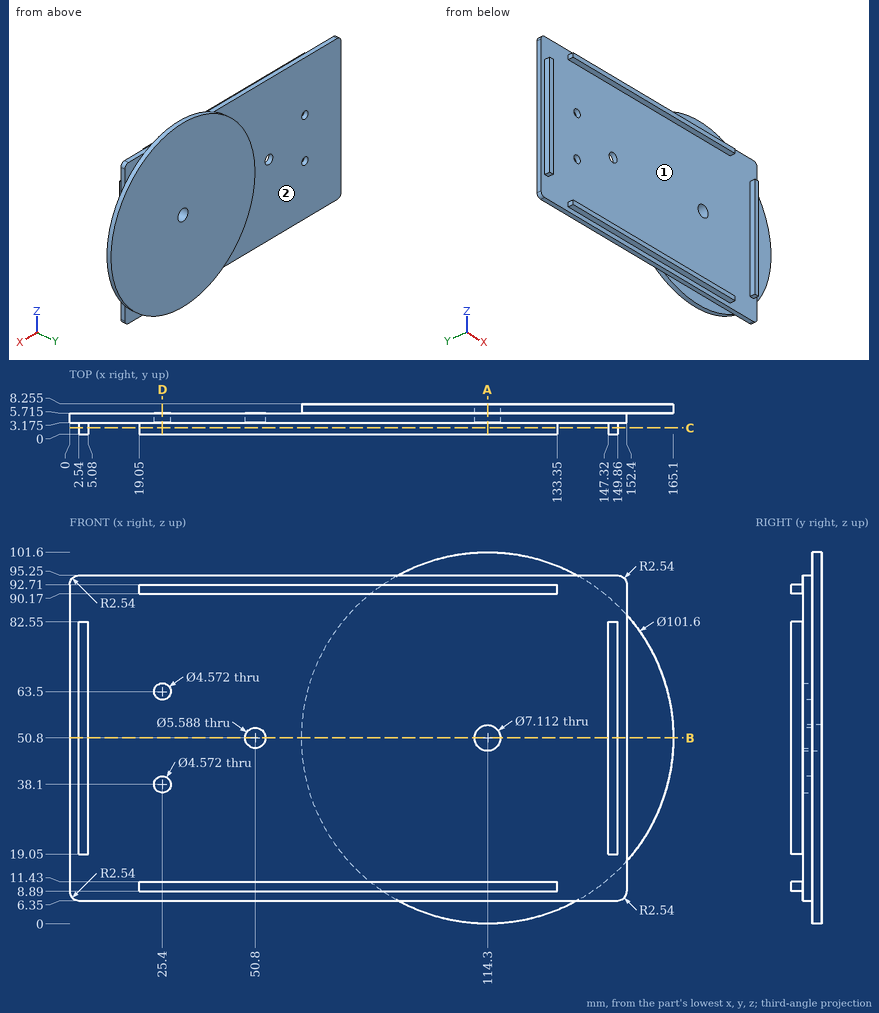
Print and shaded views of the part. All mm, measured from the part's lowest x, y and z. Round coordinates to 2 decimals unless told otherwise and drop trailing zeros. Write each loop counter-clockwise with the first axis right and the second up, starting at its lowest first coordinate (ties: lowest second). Pieces come first, ordered by that corner, then holes. Notation, with made-up numbers: (-15.75, 12.5) -> (8.25, 12.5) arc R22 ccw to (8.25, 39.5) -> close; hole circle Ø9 at (-5, -37.5). An arc over 180 degrees is marked (long way). Return JSON: item names as keys, results as strings. Group by question number.
Q1. Mould opens along Z. For the marked faces 1 and 2 say: pulls with the +Z half, pulls with the -Z half, needs draft (parallel to the pull), parting line crosses it, or undercut.
Q2. Saw through at C-C on y = 1.75. Write the cut outline in (x, z).
Q3. Probe L1, parallel to X at y = 4.25, z = 50.8; L2, parallel to Z at x = 31, y = 1.75; L3, parallel to X at y = 4.85, z = 38.1. List the from-to ranges inside material, lowest first. Write a range as [from, to].
Q4. Pin check, flat tips, straight feed: pin 1 (0.8 mm diameter, centred on y = 5, z = 52.5, fed in from +X); pin 2 (0.8 mm diameter, centred on x = 4, y = 1, fed in from +Z); pin 3 (4.5 mm diameter, centred on x = 114.3, z = 50.8, fed in from +Y); pin 4 (2 mm diameter, centred on x = 18.5, z = 34.5, fed in from +Y) (3 decimals). Stop position of each tip, or through.
Q5. Saw through at D-D on x = 25.4. Write the cut outline in (y, z) (3 decimals), plus the area to 3 significant figures.
Q6. Saw through at B-B on z = 50.8. Write the cut outline in (x, y) (3 decimals), plus the area to 3 significant figures.
Q7. Saw through at A-A on x = 114.3. Write the cut outline in (y, z) (3 decimals).
Answer:
{
 "1": {"face 1": "undercut", "face 2": "needs draft"},
 "2": {"outline": "(2.54, 19.05) -> (5.08, 19.05) -> (5.08, 82.55) -> (2.54, 82.55) -> close; (19.05, 8.89) -> (133.35, 8.89) -> (133.35, 11.43) -> (19.05, 11.43) -> close; (19.05, 90.17) -> (133.35, 90.17) -> (133.35, 92.71) -> (19.05, 92.71) -> close; (147.32, 19.05) -> (149.86, 19.05) -> (149.86, 82.55) -> (147.32, 82.55) -> close"},
 "3": {"L1": "[0, 48.01], [53.59, 110.74], [117.86, 152.4]", "L2": "[8.89, 11.43], [90.17, 92.71]", "L3": "[0, 23.11], [27.69, 152.4]"},
 "4": {"pin 1": "x = 152.4", "pin 2": "z = 82.55", "pin 3": "through", "pin 4": "y = 5.715"},
 "5": {"outline": "(0, 8.89) -> (3.175, 8.89) -> (3.175, 6.35) -> (5.715, 6.35) -> (5.715, 35.814) -> (3.175, 35.814) -> (3.175, 11.43) -> (0, 11.43) -> close; (0, 90.17) -> (3.175, 90.17) -> (3.175, 65.786) -> (5.715, 65.786) -> (5.715, 95.25) -> (3.175, 95.25) -> (3.175, 92.71) -> (0, 92.71) -> close; (3.175, 40.386) -> (5.715, 40.386) -> (5.715, 61.214) -> (3.175, 61.214) -> close", "area": "219 mm2"},
 "6": {"outline": "(0, 3.175) -> (2.54, 3.175) -> (2.54, 0) -> (5.08, 0) -> (5.08, 3.175) -> (48.006, 3.175) -> (48.006, 5.715) -> (0, 5.715) -> close; (53.594, 3.175) -> (110.744, 3.175) -> (110.744, 8.255) -> (63.5, 8.255) -> (63.5, 5.715) -> (53.594, 5.715) -> close; (117.856, 3.175) -> (147.32, 3.175) -> (147.32, 0) -> (149.86, 0) -> (149.86, 3.175) -> (152.4, 3.175) -> (152.4, 5.715) -> (165.1, 5.715) -> (165.1, 8.255) -> (117.856, 8.255) -> close", "area": "611 mm2"},
 "7": {"outline": "(0, 8.89) -> (3.175, 8.89) -> (3.175, 6.35) -> (5.715, 6.35) -> (5.715, 0) -> (8.255, 0) -> (8.255, 47.244) -> (3.175, 47.244) -> (3.175, 11.43) -> (0, 11.43) -> close; (0, 90.17) -> (3.175, 90.17) -> (3.175, 54.356) -> (8.255, 54.356) -> (8.255, 101.6) -> (5.715, 101.6) -> (5.715, 95.25) -> (3.175, 95.25) -> (3.175, 92.71) -> (0, 92.71) -> close"}
}
